```python
from build123d import *

# Parameters (mm, degrees)
SKETCH_W               = 9
SKETCH_H               = 6.5
PAD_DEPTH              = 200
SKETCH001_W            = 1
SKETCH001_H            = 0.5
POCKET_DEPTH           = 600.616776
SKETCH002_R            = 3
POCKET001_DEPTH        = 3.5
LINEARPATTERN_COUNT    = 9
LINEARPATTERN_PITCH    = 22.5
SKETCH003_R            = 1.75
POCKET002_DEPTH        = 3.001
LINEARPATTERN001_COUNT = 9
LINEARPATTERN001_PITCH = 22.5
CHAMFER_SIZE           = 0.5


with BuildPart() as part:
    # Sketch → Pad (new body)
    with BuildSketch(Plane.XY):
        with Locations((0, 3.25)):
            Rectangle(SKETCH_W, SKETCH_H)
    extrude(amount=PAD_DEPTH)

    # Sketch001 (on Face6 of Pad) → Pocket (cut, through all)
    with BuildSketch(Plane.XY.offset(200)):
        with Locations((-4, 4.5)):
            Rectangle(SKETCH001_W, SKETCH001_H)
    pocket = extrude(amount=-POCKET_DEPTH, mode=Mode.SUBTRACT)

    # Mirrored: Pocket across Sketch001 V_Axis
    add(pocket.mirror(Plane(origin=(0, 0, 200), x_dir=(0, 0, 1), z_dir=(1, 0, 0))), mode=Mode.SUBTRACT)

    # Sketch002 (on Face11 of Mirrored) → Pocket001 (cut)
    with BuildSketch(Plane(origin=(0, 6.5, 0), x_dir=(-1, 0, 0), z_dir=(0, 1, 0))):
        with Locations((0, 10)):
            Circle(SKETCH002_R)
    pocket001 = extrude(amount=-POCKET001_DEPTH, mode=Mode.SUBTRACT)

    # LinearPattern: Pocket001 ×9
    with Locations(*[(0, 0, i * LINEARPATTERN_PITCH) for i in range(1, LINEARPATTERN_COUNT)]):
        add(pocket001, mode=Mode.SUBTRACT)

    # Sketch003 (on Face31 of LinearPattern) → Pocket002 (cut, through all)
    with BuildSketch(Plane(origin=(0, 3, 0), x_dir=(-1, 0, 0), z_dir=(0, 1, 0))):
        with Locations((0, 10)):
            Circle(SKETCH003_R)
    pocket002 = extrude(amount=-POCKET002_DEPTH, mode=Mode.SUBTRACT)

    # LinearPattern001: Pocket002 ×9
    with Locations(*[(0, 0, i * LINEARPATTERN001_PITCH) for i in range(1, LINEARPATTERN001_COUNT)]):
        add(pocket002, mode=Mode.SUBTRACT)

    # Chamfer
    chamfer_edges = [part.edges().sort_by_distance(p)[0] for p in [
        (-4.5, 0, 100),
        (-4.5, 4.25, 100),
        (-4.5, 4.75, 100),
        (-4.5, 6.5, 100),
        (4.5, 0, 100),
        (4.5, 4.25, 100),
        (4.5, 4.75, 100),
        (4.5, 6.5, 100),
    ]]
    chamfer(chamfer_edges, length=CHAMFER_SIZE)


solid = part.part
```
CAD build for the part. Positions are in the model's coordinates, mm. A direction names the side the tool comes from. Round coordinates to 2 decimals unless told otherwise and drop trailing zeros. Order: outer loops, then holes, each group sorted by start corner. A loop starts at its lowest first (then second) coordinate and runs counter-clockwise, first axis right, second up. Notation, with made-up numbers: (-20.75, -21) - (2.25, -21) arc R23 cw to (2.25, 4) - close; hole circle Ø9 at (8.5, 76). An arc over 180 degrees is marked (long way). Answer in a Markdown table with one row per item. Add a question column.
(1) Band-saw the part on B-B on z = 162.5. List the corners of the cut face in (x, y).
(2) Drop a flat-ended pin along its axis: pin 1 Ø3 at (x, z) = (0, 10.5) entering from +Y. Give the stop position or say it passes through.
(3) Probe L1, parallel to Y at x = 4, z = 37.5; L2, parallel to Y at x = 2.5, z = 11; L3, parallel to X at y = 2.15, z = 77.5. List the from-to ranges inside material, lowest first. Write a range as [from, to].
(4) 3-axis set-ups, long thin cutter, end or side, ignore diameter. For faces 5 (the face through (-0.81, 1.52, 120.95)), 6 (the face through (-2, 3, 145)): which of +Z, -Z, +X, -X, +Y, -Y reach the whole face in a straight line?
(5) Band-saw the part on A-A on z = 10. List the corners of the cut face in (x, y), and give its area (3 significant figures).
(6) Mould opens along X. For faces 1 (the face through (1.29, 1.52, 146.18)), 2 (the face through (3.8, 6.5, 99.5)), 3 (the face through (-4.5, 2, 99)), 4 (the face through (4.5, 2, 99)) say: +X half, -X half, draft (parallel to the pull), parting line (faces both ways), or undercut.
Data:
| question | item | result |
|---|---|---|
| 1 | outline | (-4.5, 0.5) - (-4, 0) - (4, 0) - (4.5, 0.5) - (4.5, 3.75) - (4, 4.25) - (3.5, 4.25) - (3.5, 4.75) - (4, 4.75) - (4.5, 5.25) - (4.5, 6) - (4, 6.5) - (-4, 6.5) - (-4.5, 6) - (-4.5, 5.25) - (-4, 4.75) - (-3.5, 4.75) - (-3.5, 4.25) - (-4, 4.25) - (-4.5, 3.75) - close |
| 2 | pin 1 | stops at y = 3 |
| 3 | L1 | y = [0, 4.25], [4.75, 6.5] |
| 3 | L2 | y = [0, 3] |
| 3 | L3 | x = [-4.5, -1.75], [1.75, 4.5] |
| 4 | face 5 | +Y, -Y |
| 4 | face 6 | +Y |
| 5 | outline | (-4.5, 0.5) - (-4, 0) - (-1.75, 0) - (-1.75, 3) - (-3, 3) - (-3, 6.5) - (-4, 6.5) - (-4.5, 6) - (-4.5, 5.25) - (-4, 4.75) - (-3.5, 4.75) - (-3.5, 4.25) - (-4, 4.25) - (-4.5, 3.75) - close; (1.75, 0) - (4, 0) - (4.5, 0.5) - (4.5, 3.75) - (4, 4.25) - (3.5, 4.25) - (3.5, 4.75) - (4, 4.75) - (4.5, 5.25) - (4.5, 6) - (4, 6.5) - (3, 6.5) - (3, 3) - (1.75, 3) - close |
| 5 | area | 25.0 mm^2 |
| 6 | face 1 | undercut |
| 6 | face 2 | draft |
| 6 | face 3 | -X half |
| 6 | face 4 | +X half |
